from build123d import *

# Parameters (mm, degrees)
F2_R     = 2.3340680492
F2_R_2   = 2.3765081856
F2_R_3   = 1.2745108739
F2_R_4   = 1.1178169875
F2_R_5   = 2.3922293989
F2_R_6   = 1.767423745
F3_DEPTH = 12.7
F4_R     = 1.4997579314
F5_DEPTH = 12.7


with BuildPart() as f1:
    # F0 (on Front) → F1 (revolve)
    with BuildSketch(Plane.XZ):
        with BuildLine():
            Line((0, 101.6), (0, 88.9))
            ThreePointArc((0, 88.9), (1.3241588609, 88.9692200038), (2.6338833467, 89.1761254628))
            ThreePointArc((2.6338833467, 89.1761254628), (12.3538464369, 98.6550928344), (7.9553518202, 111.4996150136))
            Line((7.9553518202, 111.4996150136), (0, 111.4996150136))
            Line((0, 111.4996150136), (0, 101.6))
        make_face()
        with BuildLine():
            Line((0, 63.5), (0, 38.1))
            ThreePointArc((0, 38.1), (1.6292774194, 38.1523086832), (3.2518441808, 38.3090192842))
            ThreePointArc((3.2518441808, 38.3090192842), (25.3980950451, 63.8110756831), (2.6338833467, 88.7630690637))
            ThreePointArc((2.6338833467, 88.7630690637), (1.3187201717, 88.8657441663), (0, 88.9))
            Line((0, 88.9), (0, 63.5))
        make_face()
        with BuildLine():
            Line((0, 0), (0, -38.1))
            ThreePointArc((0, -38.1), (38.0652275084, -1.6274073662), (3.2518441808, 37.9609735047))
            ThreePointArc((3.2518441808, 37.9609735047), (1.6274073662, 38.0652275084), (0, 38.1))
            Line((0, 38.1), (0, 0))
        make_face()
        with BuildLine():
            ThreePointArc((0, 38.1), (1.6274073662, 38.0652275084), (3.2518441808, 37.9609735047))
            Line((3.2518441808, 37.9609735047), (3.2518441808, 38.3090192842))
            ThreePointArc((3.2518441808, 38.3090192842), (1.6292774194, 38.1523086832), (0, 38.1))
        make_face()
        with BuildLine():
            ThreePointArc((0, 88.9), (1.3187201717, 88.8657441663), (2.6338833467, 88.7630690637))
            Line((2.6338833467, 88.7630690637), (2.6338833467, 89.1761254628))
            ThreePointArc((2.6338833467, 89.1761254628), (1.3241588609, 88.9692200038), (0, 88.9))
        make_face()
    revolve(axis=Axis((0, 0, 82.55), (0, 0, 1)))

    # F2 (on Front) → F3 (join)
    with BuildSketch(Plane.XZ):
        with Locations((4.4365231879, 106.2612310052)):
            Circle(F2_R)
        with Locations((-4.890372511, 109.1067269444)):
            Circle(F2_R_2)
        with Locations((5.0688553602, 95.8277508616)):
            Circle(F2_R_3)
        with Locations((1.4329472324, 95.3535065055)):
            Circle(F2_R_4)
        with Locations((-2.361045219, 96.3020026684)):
            Circle(F2_R_5)
        with BuildLine():
            ThreePointArc((-8.8838324472, 98.8684339538), (-8.4015064273, 95.0106018582), (-5.117980782, 97.0924198627))
            ThreePointArc((-5.117980782, 97.0924198627), (-5.6877052972, 98.6083702193), (-7.1148409223, 99.3738605292))
            ThreePointArc((-7.1148409223, 99.3738605292), (-7.9210708341, 98.8472169947), (-8.8838324472, 98.8684339538))
        make_face()
        with BuildLine():
            ThreePointArc((-8.8838324472, 98.8684339538), (-7.9210708341, 98.8472169947), (-7.1148409223, 99.3738605292))
            ThreePointArc((-7.1148409223, 99.3738605292), (-8.0520311406, 99.3055776816), (-8.8838324472, 98.8684339538))
        make_face()
        with BuildLine():
            ThreePointArc((-8.8838324472, 98.8684339538), (-8.0520311406, 99.3055776816), (-7.1148409223, 99.3738605292))
            ThreePointArc((-7.1148409223, 99.3738605292), (-6.8370397391, 99.8603227191), (-6.740632268, 100.4121601582))
            ThreePointArc((-6.740632268, 100.4121601582), (-9.3194445123, 101.7328037136), (-8.8838324472, 98.8684339538))
        make_face()
        with Locations((6.8077677861, 98.6732468009)):
            Circle(F2_R_6)
    extrude(amount=F3_DEPTH)

    # F4 (on Front) → F5 (join)
    with BuildSketch(Plane.XZ):
        with Locations((0, 102.3487076163)):
            Circle(F4_R)
    extrude(amount=F5_DEPTH)


solid = f1.part
Work out the finished part from the listing and answer in its coordinate system (mm). A direction names the side the tool comes from. Give positions to 0.01 mm unless a question says otherwise; leave off trailing zeros. Loops run counter-clockwise (first coordinate to the right, second up) from the corner with the lowest first, then second, coordinate; pieces in that order, holes last. Notation, with made-up numbers: (-15.75, -30.5) -> (10.25, -30.5) arc R24 cw to (10.25, -13.5) -> close; hole circle Ø3 at (21, -17). An arc over 180 degrees is marked (long way). Use a Markdown table: item, result. Add a question column.
1. Flat-ended cylindrical pins translate along their axes: pin 1 Ø2.5 at (x, z) = (-3, 95.5) entering from -Y; pin 2 Ø3 at (y, z) = (-23, -2) entering from -X; pin 3 Ø6 at (x, z) = (13.5, -18.5) entering from -Y. Find the tip coordinate at first contact, or state that the pin passes through.
2. Section D-D on z = -6 is taken. Determine the outline of the cut face in (x, y).
3. Find the intervals of material crossed by probe 1 along Z at (x, y) = (-15, 12); probe 2 along Z at (x, y) = (-1.5, -23); probe 3 along Y at (x, z) = (4.5, 82.5), in increasing order.
4. For faces 4 (the flat face through (0, 0, 111.5)), 5 (the cylindrical face through (2.512, 0.791, 88.972)), 6 (the flat face through (-5, -12.7, 109)), determine the directions among +Z, -Z, +X, -X, +Y, -Y from which every point of the face is accessible in a straight line to the end or side of a thin tool.
5. Section B-B on x = -19 is taken. Determine the outline of the cut face in (y, z).
6. Section C-C on y = 20 is taken. Determine the outline of the cut face in (x, z), and give its area (3 significant figures).
7. Determine the mould class of faces 1 (the cylindrical face through (8.44, -11.15, 98)), 2 (the flat face through (4, -12.7, 106)), 3 (the cylindrical face through (1.501, -2.885, 38.137)) for opening direction X: released by +X, released by -X, zero draft, split by the parting line, or undercut.
8. Section A-A on y = 0 is taken. Determine the outline of the cut face in (x, z), and give its area (3 significant figures).
Results below:
| question | item | result |
|---|---|---|
| 1 | pin 1 | stops at y = -12.7 |
| 1 | pin 2 | stops at x = -31.39 |
| 1 | pin 3 | stops at y = -32.49 |
| 2 | outline | circle Ø75.25 at (0, 0) |
| 3 | probe 1 | z = -32.9 to 32.9, 46.88 to 80.12 |
| 3 | probe 2 | z = -30.34 to 30.34, 52.83 to 74.17 |
| 3 | probe 3 | y = -16.25 to 16.25 |
| 4 | face 4 | +Z, +X, -X, +Y, -Y |
| 4 | face 5 | none |
| 4 | face 6 | +Z, +X, -X, -Y |
| 5 | outline | circle Ø66.05 at (0, 0); circle Ø33.71 at (0, 63.5) |
| 6 | outline | circle Ø64.86 at (0, 0); circle Ø31.32 at (0, 63.5) |
| 6 | area | 4,070 mm^2 |
| 7 | face 1 | undercut |
| 7 | face 2 | zero draft |
| 7 | face 3 | split by the parting line |
| 8 | outline | (-7.96, 111.5) arc R12.7 ccw to (-2.63, 89.18) -> (-2.63, 88.76) arc R25.4 ccw to (-3.25, 38.31) -> (-3.25, 37.96) arc R38.1 ccw (long way) to (3.25, 37.96) -> (3.25, 38.31) arc R25.4 ccw to (2.63, 88.76) -> (2.63, 89.18) arc R12.7 ccw to (7.96, 111.5) -> close |
| 8 | area | 7,060 mm^2 |
